Check sheet for the modelled part. Datum: model origin and axes. Units: mm. A direction names the side the tool comes from. Give positions to 0.01 mm unless a question says otherwise; leave off trailing zeros. Order: outer loops, then holes, each group sorted by start corner. A loop starts at its lowest first (then second) coordinate and runs counter-clockwise, first axis right, second up. Notation, with made-up numbers: M 36,-16.5 L 87,-16.5 A31 ccw 87,21.5 Z; hole C 88.5,-28.75 d2. An arc over 180 degrees is marked long. One line per question, with ' | ' between items. Start each with the question number.
```python
from build123d import *

# Parameters (mm, degrees)
BOSS_EXTRUDE1_DEPTH = 2.5
FILLET1_R           = 1


with BuildPart() as part:
    # Sketch1 → Boss-Extrude1 (new body)
    with BuildSketch(Plane(origin=(0, 0, 0), x_dir=(1, 0, 0), z_dir=(0, 1, 0))):
        Polygon((0, 0), (42.5, 35), (95, 45), (70, 0), (70, -1.8), (45, -1.8), (45, 0), (30, 0), (30, -1.8), (5, -1.8), (5, 0), align=None)
    extrude(amount=BOSS_EXTRUDE1_DEPTH)

    # Fillet1
    fillet1_edges = [part.edges().sort_by_distance(p)[0] for p in [
        (21.25, 0, -17.5),
        (68.75, 0, -40),
        (42.5, 1.25, -35),
        (68.75, 2.5, -40),
        (21.25, 2.5, -17.5),
    ]]
    fillet(fillet1_edges, radius=FILLET1_R)


solid = part.part
```
Item 1: Go/stop test with flat-tipped pins: P1, Ø1.5, axis at x = 48, y = 1, coming from the -Z side; P2, Ø0.9, axis at y = 1, z = 1, coming from the +X side; P3, Ø0.9, axis at y = 1.5, z = 0.5, coming from the -X side; P4, Ø3, axis at x = 27.5, z = -22.5, coming from the +Y side. Record where each tip stops, or that it passes through.
Item 2: Scan lines: probe 1 along X at (y, z) = (2, -15); probe 2 along X at (y, z) = (0.95, -13); probe 3 along Z at (x, y) = (81, 2.15). Record each from-to range of solid material in increasing order. Write a range as [from, to].
Item 3: Draft check along X on faces 4 (the face through (68.51, 1.246, -39.954)), 5 (the face through (38, 1, 0)), 6 (the face through (82.675, 1.232, -22.815)), 7 (the face through (45, 1, 1)). Enter one of: released by +X, released by -X, zero draft, split by the parting line, or undercut.
Item 4: Set-up check for faces 1 (the face through (3, 1, 0)), 2 (the face through (70, 1, 1)), 3 (the face through (30, 1, 1)): record each of +Z, -Z, +X, -X, +Y, -Y from which the full face is reachable in a straight line by a thin tool's end or side.
Item 5: Section check A-A, the plane y = 0.4. Record the cut outline in (x, z).
Reported:
1) P1: stops at z = -36.19 | P2: stops at x = 70 | P3: stops at x = 5 | P4: stops at y = 2.5
2) probe 1: x = [18.43, 78.33] | probe 2: x = [15.79, 77.22] | probe 3: z = [-42.09, -19.8]
3) face 4: released by -X | face 5: undercut | face 6: released by +X | face 7: undercut
4) face 1: +Z, -X, +Y, -Y | face 2: +Z, +X, +Y, -Y | face 3: +Z, +Y, -Y
5) outline: M 0.31,0 L 42.43,-34.68 A0.8 ccw 42.79,-34.85 L 94.87,-44.77 L 70,0 L 70,1.8 L 45,1.8 L 45,0 L 30,0 L 30,1.8 L 5,1.8 L 5,0 Z
